Verification items for the finished model (mm, model axes). Face numbers are marked on the shaded views. Round coordinates to 2 decimals unless told otherwise and drop trailing zeros. Write each loop counter-clockwise with the first axis right and the second up, starting at its lowest first coordinate (ties: lowest second). Pieces come first, ordered by that corner, then holes. Notation, with made-up numbers: (30, -11.75) -> (63, -11.75) arc R36 ccw to (63, 26.25) -> close; hole circle Ø5 at (-25, -30.75). An arc over 180 degrees is marked (long way). Use CSV: the item, a comma, the result in double quotes.
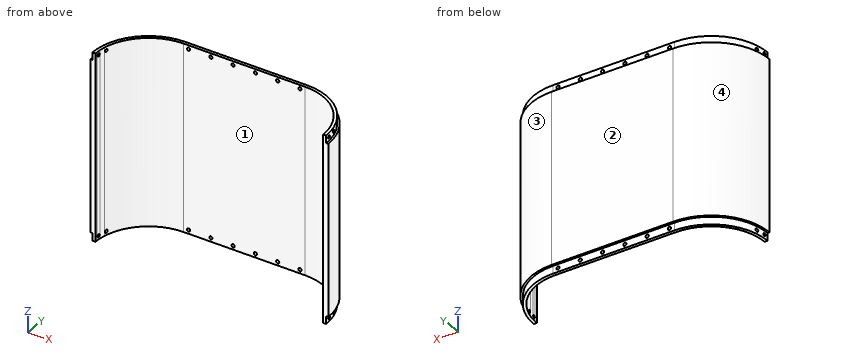
```python
from build123d import *

# Parameters (mm, degrees)
BOSS_EXTRUDE1_DEPTH = 92.5
SKETCH2_R           = 1.5
CUT_EXTRUDE1_DEPTH  = 161.2146997
SKETCH4_R           = 1.6
CUT_EXTRUDE2_DEPTH  = 161.214699867
CUT_EXTRUDE3_DEPTH  = 7.5


with BuildPart() as part:
    # Sketch1 → Boss-Extrude1 (new, symmetric)
    with BuildSketch(Plane.XY):
        with BuildLine():
            ThreePointArc((117.5, 0), (100.658639918, 40.658639918), (60, 57.5))
            Line((60, 57.5), (-60, 57.5))
            ThreePointArc((-60, 57.5), (-100.658639918, 40.658639918), (-117.5, 0))
            Line((-117.5, 0), (-112.5, 0))
            ThreePointArc((-112.5, 0), (-112.485698596, 1.22533379), (-112.442802175, 2.45))
            ThreePointArc((-112.442802175, 2.45), (-112.306489538, 4.503460029), (-112.089802265, 6.55))
            ThreePointArc((-112.089802265, 6.55), (-111.721057974, 9.010114432), (-111.236193262, 11.45))
            ThreePointArc((-111.236193262, 11.45), (-110.731665892, 13.511035335), (-110.144266871, 15.55))
            ThreePointArc((-110.144266871, 15.55), (-91.143819612, 42.264790311), (-60, 52.5))
            Line((-60, 52.5), (-57.05, 52.5))
            Line((-57.05, 52.5), (-52.95, 52.5))
            Line((-52.95, 52.5), (-35.05, 52.5))
            Line((-35.05, 52.5), (-30.95, 52.5))
            Line((-30.95, 52.5), (-13.05, 52.5))
            Line((-13.05, 52.5), (-8.95, 52.5))
            Line((-8.95, 52.5), (8.95, 52.5))
            Line((8.95, 52.5), (13.05, 52.5))
            Line((13.05, 52.5), (30.95, 52.5))
            Line((30.95, 52.5), (35.05, 52.5))
            Line((35.05, 52.5), (52.95, 52.5))
            Line((52.95, 52.5), (57.05, 52.5))
            Line((57.05, 52.5), (60, 52.5))
            ThreePointArc((60, 52.5), (91.143819612, 42.264790311), (110.144266871, 15.55))
            ThreePointArc((110.144266871, 15.55), (110.731665892, 13.511035335), (111.236193262, 11.45))
            ThreePointArc((111.236193262, 11.45), (111.721057974, 9.010114432), (112.089802265, 6.55))
            ThreePointArc((112.089802265, 6.55), (112.306489538, 4.503460029), (112.442802175, 2.45))
            ThreePointArc((112.442802175, 2.45), (112.485698596, 1.22533379), (112.5, 0))
            Line((112.5, 0), (117.5, 0))
        make_face()
    extrude(amount=BOSS_EXTRUDE1_DEPTH, both=True)

    # Sketch2 → Cut-Extrude1 (cut, symmetric)
    with BuildSketch(Plane(origin=(0, 0, 0), x_dir=(0, 0, -1), z_dir=(1, 0, 0))):
        with Locations((-88.75, 4.5)):
            Circle(SKETCH2_R)
        with Locations((-88.75, 13.5)):
            Circle(SKETCH2_R)
    cut_extrude1 = extrude(amount=CUT_EXTRUDE1_DEPTH, both=True, mode=Mode.SUBTRACT)

    # Sketch4 → Cut-Extrude2 (cut, symmetric)
    with BuildSketch(Plane(origin=(0, 57.5, 0), x_dir=(1, 0, 0), z_dir=(0, 1, 0))):
        with Locations(Location((-55, -88.75, 0), (0, 0, 270))):
            Circle(SKETCH4_R)
        with Locations(Location((-33, -88.75, 0), (0, 0, 270))):
            Circle(SKETCH4_R)
        with Locations(Location((-11, -88.75, 0), (0, 0, 270))):
            Circle(SKETCH4_R)
        with Locations(Location((11, -88.75, 0), (0, 0, 270))):
            Circle(SKETCH4_R)
        with Locations(Location((33, -88.75, 0), (0, 0, 270))):
            Circle(SKETCH4_R)
        with Locations(Location((55, -88.75, 0), (0, 0, 270))):
            Circle(SKETCH4_R)
    cut_extrude2 = extrude(amount=CUT_EXTRUDE2_DEPTH, both=True, mode=Mode.SUBTRACT)

    # Sketch5 → Cut-Extrude3 (cut)
    with BuildSketch(Plane(origin=(0, 0, -92.5), x_dir=(-1, 0, 0), z_dir=(0, 0, -1))):
        with BuildLine():
            Line((115.5, 0), (117.5, 0))
            ThreePointArc((117.5, 0), (100.658639918, 40.658639918), (60, 57.5))
            Line((60, 57.5), (-60, 57.5))
            ThreePointArc((-60, 57.5), (-100.658639918, 40.658639918), (-117.5, 0))
            Line((-117.5, 0), (-115.5, 0))
            ThreePointArc((-115.5, 0), (-99.244426356, 39.244426356), (-60, 55.5))
            Line((-60, 55.5), (60, 55.5))
            ThreePointArc((60, 55.5), (99.244426356, 39.244426356), (115.5, 0))
        make_face()
    cut_extrude3 = extrude(amount=-CUT_EXTRUDE3_DEPTH, mode=Mode.SUBTRACT)

    # Mirror1: Cut-Extrude1, Cut-Extrude2, Cut-Extrude3 across plane
    add(cut_extrude1.mirror(Plane.XY), mode=Mode.SUBTRACT)
    add(cut_extrude2.mirror(Plane.XY), mode=Mode.SUBTRACT)
    add(cut_extrude3.mirror(Plane.XY), mode=Mode.SUBTRACT)


solid = part.part
```
Q1. Material ranges on L1, parallel to Z at x = 114.35, y = 4.5; L2, parallel to Y at x = -57, z = -26.5; L3, parallel to X at y = 24, z = -15, recorded low to high.
Filled in:
L1,"-92.5 to -90.25, -87.25 to 87.25, 90.25 to 92.5"
L2,"52.5 to 57.5"
L3,"-112.25 to -106.69, 106.69 to 112.25"
Q2. Section check B-B (x = 44.5). Record the cut outline in (y, z), plus the area to 3 significant figures.
Filled in:
outline,"(52.5, -92.5) -> (55.5, -92.5) -> (55.5, -85) -> (57.5, -85) -> (57.5, 85) -> (55.5, 85) -> (55.5, 92.5) -> (52.5, 92.5) -> close"
area,"895 mm²"
Q3. Mould release check, pull along X, two halves, no side actions. Record for the marked faces 1, 2, 3 and 4: released by +X, released by -X, zero draft, split by the parting line, or undercut.
Filled in:
face 1,"undercut"
face 2,"zero draft"
face 3,"released by +X"
face 4,"released by -X"
Q4. Section check C-C (z = -46). Record the cut outline in (x, y).
Filled in:
outline,"(-117.5, 0) -> (-112.5, 0) arc R52.5 cw to (-60, 52.5) -> (60, 52.5) arc R52.5 cw to (112.5, 0) -> (117.5, 0) arc R57.5 ccw to (60, 57.5) -> (-60, 57.5) arc R57.5 ccw to start"
Q5. Section check A-A (y = 41). Record the cut outline in (x, z).
Filled in:
outline,"(-100.31, -85) -> (-97.41, -85) -> (-97.41, -92.5) -> (-92.79, -92.5) -> (-92.79, 92.5) -> (-97.41, 92.5) -> (-97.41, 85) -> (-100.31, 85) -> close; (92.79, -92.5) -> (97.41, -92.5) -> (97.41, -85) -> (100.31, -85) -> (100.31, 85) -> (97.41, 85) -> (97.41, 92.5) -> (92.79, 92.5) -> close"
Q6. Section check D-D (y = 22.5). Record the cut outline in (x, z), plus the area to 3 significant figures.
Filled in:
outline,"(-112.92, -85) -> (-110.73, -85) -> (-110.73, -92.5) -> (-107.43, -92.5) -> (-107.43, 92.5) -> (-110.73, 92.5) -> (-110.73, 85) -> (-112.92, 85) -> close; (107.43, -92.5) -> (110.73, -92.5) -> (110.73, -85) -> (112.92, -85) -> (112.92, 85) -> (110.73, 85) -> (110.73, 92.5) -> (107.43, 92.5) -> close"
area,"1,960 mm²"
Q7. Go/stop test with flat-tipped pins: P1, Ø1.8, axis at y = 13.5, z = -88.75, coming from the +X side (3 decimals); P2, Ø5, axis at x = 55, z = -88.75, coming from the +Y side; P3, Ø4, axis at y = 43, z = -71, coming from the -X side; P4, Ø10, axis at y = 14.5, z = 69, coming from the +X side. Record where each tip stops, or that it passes through.
Filled in:
P1,"through"
P2,"y = 55.5"
P3,"x = -100.31"
P4,"x = 116.71"
